Source: CAD feature listing. Evaluate the final solid. Frame: model axes, mm. A direction names the side the tool comes from. Round coordinates to 2 decimals unless told otherwise and drop trailing zeros. Order: outer loops, then holes, each group sorted by start corner. A loop starts at its lowest first (then second) coordinate and runs counter-clockwise, first axis right, second up. Notation, with made-up numbers: (-6, 16.25) - (49, 16.25) arc R19 ccw to (49, 24.25) - close; hole circle Ø11 at (-20.5, 23). An arc over 180 degrees is marked (long way). Put each result on its own line as item: value. Start each with the question number.
1) Access query for faces 4 (the face through (-24, -36, -2.588)), 5 (the face through (-36.255, 29.336, -5.435)). Directions: +Z, -Z, +X, -X, +Y, -Y. A direction counts if a zero-diameter tool reaches every point of the face in a straight line with its end or side. Return the directions, or none.
2) Contact query for flat-ended pins moving along their axis: P1, Ø1.2, axis at x = -8, y = 5, coming from the +Z side; P2, Ø18.5, axis at x = 28.28, y = -28.28, coming from the +Z side; P3, Ø1.5, axis at x = -38, y = 16.5, coming from the +Z side. Output: stop coordinate, or through.
3) Section A-A on z = 11.5. Output: boundary loops of the cut face in (x, y) (3 decimals), then the cut area to 3 significant figures.
4) Section B-B on y = 0. State how many separate pieces and enclosed holes the cut face has, then the cut area to 3 significant figures.
5) Line query: probe 1 along Y at (x, z) = (0, 14.5) (3 decimals); probe 2 along Y at (x, z) = (0, -0.6); probe 3 along X at (y, z) = (36.5, -2.5). Output: solid intervals per line, ascending. Write a range as [from, to].
6) Mould query, pull axis X, two halves, no side actions, for faces 1 (the face through (-1, -14, -7.85)), 2 (the face through (2.6, -7.2, -0.85)), 3 (the face through (4.444, -20.013, -0.493)). Classes: +X half, -X half, draft (parallel to the pull), parting line (faces both ways), or undercut.
7) Section C-C on z = 3. Output: boundary loops of the cut face in (x, y), then the cut area to 3 significant figures.
```python
from build123d import *

# Parameters (mm, degrees)
SKETCH1_R                    = 17.45
BOSS_EXTRUDE1_DEPTH          = 19
SKETCH7_R                    = 20.5
BOSS_EXTRUDE3_DEPTH          = 1
SKETCH3_R                    = 57.5
BOSS_EXTRUDE2_DEPTH          = 6.85
SKETCH4_R                    = 11.075
CUT_EXTRUDE1_DEPTH           = 7
SKETCH5_R                    = 7.5
CUT_EXTRUDE2_DEPTH           = 0.5
SKETCH6_R                    = 2.025
CUT_EXTRUDE3_DEPTH           = 10
CIRPATTERN1_COUNT            = 6
CHAMFER1_SIZE                = 1
SKETCH8_R                    = 8.04
CUT_EXTRUDE4_DEPTH           = 84.740671122
SKETCH9_R                    = 11.2125
CUT_EXTRUDE5_DEPTH           = 1.5875
CHAMFER2_SIZE                = 0.5
CHAMFER3_SIZE                = 0.5
CIRPATTERN2_COUNT            = 8
CHAMFER2_OF_CIRPATTERN2_SIZE = 0.5
CHAMFER3_OF_CIRPATTERN2_SIZE = 0.5


with BuildPart() as part:
    # Sketch1 → Boss-Extrude1 (new body)
    with BuildSketch(Plane.XY):
        Circle(SKETCH1_R)
    extrude(amount=BOSS_EXTRUDE1_DEPTH)

    # Sketch7 → Boss-Extrude3 (add)
    with BuildSketch(Plane(origin=(0, 0, 0), x_dir=(-1, 0, 0), z_dir=(0, 0, -1))):
        Circle(SKETCH7_R)
    extrude(amount=BOSS_EXTRUDE3_DEPTH)

    # Sketch3 → Boss-Extrude2 (add)
    with BuildSketch(Plane(origin=(0, 0, -1), x_dir=(-1, 0, 0), z_dir=(0, 0, -1))):
        with Locations(Location((0, 0, 0), (0, 0, 180))):
            Circle(SKETCH3_R)
    extrude(amount=BOSS_EXTRUDE2_DEPTH)

    # Sketch4 → Cut-Extrude1 (cut)
    with BuildSketch(Plane(origin=(0, 0, -7.85), x_dir=(-1, 0, 0), z_dir=(0, 0, -1))):
        Circle(SKETCH4_R)
    extrude(amount=-CUT_EXTRUDE1_DEPTH, mode=Mode.SUBTRACT)

    # Sketch5 → Cut-Extrude2 (cut)
    with BuildSketch(Plane(origin=(0, 0, -0.85), x_dir=(-1, 0, 0), z_dir=(0, 0, -1))):
        Circle(SKETCH5_R)
    extrude(amount=-CUT_EXTRUDE2_DEPTH, mode=Mode.SUBTRACT)

    # Sketch6 → Cut-Extrude3 (cut)
    with BuildSketch(Plane.XY.offset(19)):
        with Locations((0, 10)):
            Circle(SKETCH6_R)
    cut_extrude3 = extrude(amount=-CUT_EXTRUDE3_DEPTH, mode=Mode.SUBTRACT)

    # CirPattern1: Cut-Extrude3 ×6 about axis
    cirpattern1_axis = Axis((0, 0, 0), (0, 0, 1))
    for i in range(1, CIRPATTERN1_COUNT):
        add(cut_extrude3.rotate(cirpattern1_axis, i * 360 / CIRPATTERN1_COUNT), mode=Mode.SUBTRACT)

    # Chamfer1
    chamfer1_edges = [part.edges().sort_by_distance(p)[0] for p in [
        (11.075, 0, -7.85),
        (-17.45, 0, 19),
    ]]
    chamfer(chamfer1_edges, length=CHAMFER1_SIZE)

    # Sketch8 → Cut-Extrude4 (cut, through all)
    with BuildSketch(Plane.XY.offset(-1)):
        with Locations((-40, 0)):
            Circle(SKETCH8_R)
    cut_extrude4 = extrude(amount=-CUT_EXTRUDE4_DEPTH, mode=Mode.SUBTRACT)

    # Sketch9 → Cut-Extrude5 (cut)
    with BuildSketch(Plane.XY.offset(-1)):
        with Locations((-40, 0)):
            Circle(SKETCH9_R)
    cut_extrude5 = extrude(amount=-CUT_EXTRUDE5_DEPTH, mode=Mode.SUBTRACT)

    # Chamfer2
    chamfer2_edges = [part.edges().sort_by_distance(p)[0] for p in [
        (-48.04, 0, -2.5875),
    ]]
    chamfer(chamfer2_edges, length=CHAMFER2_SIZE)

    # Chamfer3
    chamfer3_edges = [part.edges().sort_by_distance(p)[0] for p in [
        (-51.2125, 0, -1),
    ]]
    chamfer(chamfer3_edges, length=CHAMFER3_SIZE)

    # CirPattern2: Cut-Extrude4, Cut-Extrude5 ×8 about axis
    cirpattern2_axis = Axis((0, 0, 0), (0, 0, 1))
    add([cut_extrude4.rotate(cirpattern2_axis, i * 360 / CIRPATTERN2_COUNT) for i in range(1, CIRPATTERN2_COUNT)], mode=Mode.SUBTRACT)
    add([cut_extrude5.rotate(cirpattern2_axis, i * 360 / CIRPATTERN2_COUNT) for i in range(1, CIRPATTERN2_COUNT)], mode=Mode.SUBTRACT)

    # Chamfer2 of CirPattern2
    chamfer2_of_cirpattern2_edges = [part.edges().sort_by_distance(p)[0] for p in [
        (-33.969409768, -33.969409768, -2.5875),
        (0, -48.04, -2.5875),
        (33.969409768, -33.969409768, -2.5875),
        (48.04, 0, -2.5875),
        (33.969409768, 33.969409768, -2.5875),
        (0, 48.04, -2.5875),
        (-33.969409768, 33.969409768, -2.5875),
    ]]
    chamfer(chamfer2_of_cirpattern2_edges, length=CHAMFER2_OF_CIRPATTERN2_SIZE)

    # Chamfer3 of CirPattern2
    chamfer3_of_cirpattern2_edges = [part.edges().sort_by_distance(p)[0] for p in [
        (-36.212706032, -36.212706032, -1),
        (0, -51.2125, -1),
        (36.212706032, -36.212706032, -1),
        (51.2125, 0, -1),
        (36.212706032, 36.212706032, -1),
        (0, 51.2125, -1),
        (-36.212706032, 36.212706032, -1),
    ]]
    chamfer(chamfer3_of_cirpattern2_edges, length=CHAMFER3_OF_CIRPATTERN2_SIZE)


solid = part.part
```
Answer sheet:
1. face 4: +Z
1. face 5: +Z, -Z
2. P1: z = 9
2. P2: z = -2.59
2. P3: z = -1
3. outline: circle Ø34.9 at (0, 0); hole circle Ø4.05 at (-8.66, -5); hole circle Ø4.05 at (-8.66, 5); hole circle Ø4.05 at (0, -10); hole circle Ø4.05 at (0, 10); hole circle Ø4.05 at (8.66, -5); hole circle Ø4.05 at (8.66, 5)
3. area: 879 mm^2
4. separate pieces: 3
4. enclosed holes: 0
4. area: 1,090 mm^2
5. probe 1: [-17.45, -12.025], [-7.975, 7.975], [12.025, 17.45]
5. probe 2: [-20.5, -7.5], [7.5, 20.5]
5. probe 3: [-44.43, -35.91], [-20.65, -10.65], [10.65, 20.65], [35.91, 44.43]
6. face 1: draft
6. face 2: undercut
6. face 3: parting line
7. outline: circle Ø34.9 at (0, 0)
7. area: 957 mm^2
